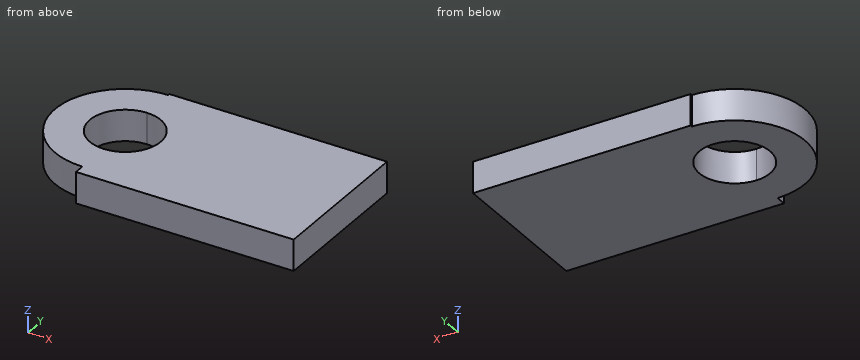
```python
from build123d import *

# Parameters (mm, degrees)
F1_DEPTH = 12.7


with BuildPart() as f1:
    # F0 (on Top) → F1 (new body)
    with BuildSketch(Plane.XY):
        with BuildLine():
            Line((-44.3014800549, -32.8442007303), (44.3014800549, -32.8442007303))
            Line((44.3014800549, -32.8442007303), (44.3014800549, 29.407016933))
            Line((44.3014800549, 29.407016933), (-44.3014800549, 29.407016933))
            Line((-44.3014800549, 29.407016933), (-44.3014800549, 28.5903187115))
            ThreePointArc((-44.3014800549, 28.5903187115), (-24.0850718176, 20.2164082372), (-15.7111613433, 0))
            ThreePointArc((-15.7111613433, 0), (-24.0850718176, -20.2164082372), (-44.3014800549, -28.5903187115))
            Line((-44.3014800549, -28.5903187115), (-44.3014800549, -32.8442007303))
        make_face()
        with BuildLine():
            ThreePointArc((-44.3014800549, 28.5903187115), (-72.8917987664, 0), (-44.3014800549, -28.5903187115))
            Line((-44.3014800549, -28.5903187115), (-44.3014800549, -14.4344542652))
            ThreePointArc((-44.3014800549, -14.4344542652), (-58.73593432, 0), (-44.3014800549, 14.4344542652))
            Line((-44.3014800549, 14.4344542652), (-44.3014800549, 28.5903187115))
        make_face()
        with BuildLine():
            Line((-44.3014800549, -14.4344542652), (-44.3014800549, -28.5903187115))
            ThreePointArc((-44.3014800549, -28.5903187115), (-24.0850718176, -20.2164082372), (-15.7111613433, 0))
            ThreePointArc((-15.7111613433, 0), (-24.0850718176, 20.2164082372), (-44.3014800549, 28.5903187115))
            Line((-44.3014800549, 28.5903187115), (-44.3014800549, 14.4344542652))
            ThreePointArc((-44.3014800549, 14.4344542652), (-34.0947795612, 10.2067004936), (-29.8670257897, 0))
            ThreePointArc((-29.8670257897, 0), (-34.0947795612, -10.2067004936), (-44.3014800549, -14.4344542652))
        make_face()
    extrude(amount=F1_DEPTH)


solid = f1.part
```
Check sheet for the modelled part. Datum: model origin and axes. Units: mm. Round coordinates to 2 decimals unless told otherwise and drop trailing zeros. Order: outer loops, then holes, each group sorted by start corner. A loop starts at its lowest first (then second) coordinate and runs counter-clockwise, first axis right, second up. Notation, with made-up numbers: (78, 16.5) - (83, 16.5) arc R27 ccw to (83, 51.5) - close; hole circle Ø11 at (61.25, 29). An arc over 180 degrees is marked (long way). Write item = value, one per line.
Q1. Section check A-A (y = 0). Record the boundary of the cut face in (x, z).
Computed:
outline = (-72.89, 0) - (-58.74, 0) - (-58.74, 12.7) - (-72.89, 12.7) - close; (-29.87, 0) - (44.3, 0) - (44.3, 12.7) - (-29.87, 12.7) - close
Q2. Section check C-C (y = 6.5). Record the boundary of the cut face in (x, z).
Computed:
outline = (-72.14, 0) - (-57.19, 0) - (-57.19, 12.7) - (-72.14, 12.7) - close; (-31.41, 0) - (44.3, 0) - (44.3, 12.7) - (-31.41, 12.7) - close
Q3. Go/stop test with flat-tipped pins: pin 1 (1 mm diameter, centred on x = 3.5, y = 6.5, fed in from -Z); pin 2 (3 mm diameter, centred on y = -3, z = 9, fed in from -X); pin 3 (5 mm diameter, centred on y = -19, z = 1.5, fed in from -X); pin 4 (3.5 mm diameter, centred on y = -31.5, z = 9, fed in from -X). Record where each tip stops, or that it passes through.
Computed:
pin_1 = 0
pin_2 = -72.85
pin_3 = -67.65
pin_4 = -44.3
Q4. Thickness scan on line 1 along X through (y, z) = (8.5, 9.25); line 2 along X through (y, z) = (11, 5.5); line 3 along X through (y, z) = (-29, 3.5). Record the ranges inside material, lowest first.
Computed:
line_1 = -71.6 to -55.97, -32.64 to 44.3
line_2 = -70.69 to -53.65, -34.96 to 44.3
line_3 = -44.3 to 44.3
Q5. Section check B-B (z = 8.25). Record the boundary of the cut face in (x, y).
Computed:
outline = (-44.3, -32.84) - (44.3, -32.84) - (44.3, 29.41) - (-44.3, 29.41) - (-44.3, 28.59) arc R28.59 ccw to (-44.3, -28.59) - close; hole circle Ø28.87 at (-44.3, 0)
Q6. Section check D-D (y = 18). Record the boundary of the cut face in (x, z).
Computed:
outline = (-66.51, 0) - (44.3, 0) - (44.3, 12.7) - (-66.51, 12.7) - close
